from build123d import *
from build123d.topology import SkipClean

# Parameters (mm, degrees)
BASPROSKE_W         = 10
BASPROSKE_H         = 15
TOOTHCUT_DEPTH      = 24.452078799
TEETHCUTS_COUNT     = 28
TEETHCUTS_ANGLE     = 347.142857143
BORSKE_R            = 3.3
BORE_DEPTH          = 50.0000508
SKETCH_1_R          = 15
CUT_EXTRUDE_1_DEPTH = 6
CUT_EXTRUDE_2_DEPTH = 10
SKETCH_3_R          = 1.8
CUT_EXTRUDE_3_DEPTH = 10


with BuildPart() as part:
    # BasProSke → Base-Revolve (revolve)
    with BuildSketch(Plane(origin=(0, 0, 0), x_dir=(1, 0, 0), z_dir=(0, 1, 0)), mode=Mode.PRIVATE) as base_revolve_sk:
        with Locations((5, 7.5)):
            Rectangle(BASPROSKE_W, BASPROSKE_H)
    revolve(base_revolve_sk.sketch.rotate(Axis((-10, 0, 0), (1, 0, 0)), 180), axis=Axis((-10, 0, 0), (1, 0, 0)))

    # TooCutSke → ToothCut (cut, through all)
    with BuildSketch(Plane(origin=(0, 0, 0), x_dir=(0, 0, -1), z_dir=(1, 0, 0))):
        with BuildLine():
            ThreePointArc((0.471336039, 12.740284272), (0, 12.749), (-0.471336039, 12.740284272))
            ThreePointArc((-0.471336039, 12.740284272), (-0.81983923, 13.900763331), (-1.409805137, 14.959114099))
            ThreePointArc((-1.409805137, 14.959114099), (0, 15.0254), (1.409805137, 14.959114099))
            ThreePointArc((1.409805137, 14.959114099), (0.81983923, 13.900763331), (0.471336039, 12.740284272))
        make_face()
    toothcut = extrude(amount=TOOTHCUT_DEPTH, mode=Mode.SUBTRACT)

    # TeethCuts: ToothCut ×28 about axis
    teethcuts_axis = Axis((-10, 0, 0), (1, 0, 0))
    for i in range(1, TEETHCUTS_COUNT):
        add(toothcut.rotate(teethcuts_axis, i * TEETHCUTS_ANGLE / (TEETHCUTS_COUNT - 1)), mode=Mode.SUBTRACT)

    # BorSke → Bore (cut, symmetric)
    with BuildSketch(Plane(origin=(0, 0, 0), x_dir=(0, 0, -1), z_dir=(1, 0, 0))):
        with Locations(Location((0, 0, 0), (0, 0, 180))):
            Circle(BORSKE_R)
    extrude(amount=BORE_DEPTH, both=True, mode=Mode.SUBTRACT)

    # ｽｹｯﾁ1 → ｶｯﾄ - 押し出し1 (cut)
    with BuildSketch(Plane(origin=(10, 0, 0), x_dir=(0, 0, -1), z_dir=(1, 0, 0))):
        Circle(SKETCH_1_R)
    extrude(amount=-CUT_EXTRUDE_1_DEPTH, mode=Mode.SUBTRACT)

    # ｽｹｯﾁ2 → ｶｯﾄ - 押し出し2 (cut)
    with SkipClean():  # the faces are left unmerged after this step: merging them gives an invalid solid
        with BuildSketch(Plane.ZY):
            with BuildLine():
                Line((-12.525740882, -2.375461295), (-14.737321612, -2.794879553))
                ThreePointArc((-14.737321612, -2.794879553), (-6.004168657, 13.745906981), (12.065215177, 8.912383672))
                Line((12.065215177, 8.912383672), (10.254628553, 7.574931963))
                ThreePointArc((10.254628553, 7.574931963), (-5.10314308, 11.68310454), (-12.525740882, -2.375461295))
            make_face()
        extrude(amount=-CUT_EXTRUDE_2_DEPTH, mode=Mode.SUBTRACT)

    # ｽｹｯﾁ3 → ｶｯﾄ - 押し出し3 (cut)
    with SkipClean():  # the faces are left unmerged after this step: merging them gives an invalid solid
        with BuildSketch(Plane(origin=(4, 0, 0), x_dir=(0, 0, -1), z_dir=(1, 0, 0))):
            with Locations((-6.885831114, 1.259098832)):
                Circle(SKETCH_3_R)
            with Locations((1.259098832, 6.885831114)):
                Circle(SKETCH_3_R)
            with Locations((6.885831114, -1.259098832)):
                Circle(SKETCH_3_R)
            with Locations((-1.259098832, -6.885831114)):
                Circle(SKETCH_3_R)
        extrude(amount=-CUT_EXTRUDE_3_DEPTH, mode=Mode.SUBTRACT)


solid = part.part
Check sheet for the modelled part. Datum: model origin and axes. Units: mm. A direction names the side the tool comes from. Round coordinates to 2 decimals unless told otherwise and drop trailing zeros. Write each loop counter-clockwise with the first axis right and the second up, starting at its lowest first coordinate (ties: lowest second). Pieces come first, ordered by that corner, then holes. Notation, with made-up numbers: (5.25, 57.5) -> (37.25, 57.5) arc R17 ccw to (37.25, 87.5) -> close; hole circle Ø4 at (5.25, 19.25). An arc over 180 degrees is marked (long way). Answer as CSV lines item,"result". Start each with the question number.
1) Go/stop test with flat-tipped pins: P1, Ø1.5, axis at x = 1, y = -4.5, coming from the +Z side; P2, Ø3, axis at y = -1.26, z = -6.89, coming from the -X side; P3, Ø1.5, axis at x = 3, y = -0.5, coming from the +Z side. Record where each tip stops, or that it passes through.
2) Section check A-A on y = 0. Enter the section's corners in (x, z), and give its area (3 significant figures).
3) Release check for a two-part mould opening along Y. For faces 1 (the cylindrical face through (2, 2.3, 13.7)), 2 (the flat face through (4, -1, 4)), 3 (the cylindrical face through (1.972, -13.872, -0.808)) record: pulls with the +Y half, pulls with the -Y half, needs draft (parallel to the pull), parting line crosses it, or undercut.
4) Tool access check on faces 4 (the flat face through (0, -1, 4)), 5 (the cylindrical face through (2, -11.5, -5.5)), 6 (the cylindrical face through (1.972, -3.894, -13.372)), 7 (the cylindrical face through (1.97, -12.75, 0.01)), 8 (the cylindrical face through (1.97, -2.83, 12.43)). Record the directions out of +Z, -Z, +X, -X, +Y, -Y that give a thin tool (end or side, any length) a straight path to the whole face; none if there is none.
5) Section check C-C on x = 1.55. State how many separate pieces and enclosed holes the cut face has, and give its area (3 significant figures).
6) Material ranges on line 1 (Y direction, x = 2.1, z = -1.25); line 2 (Y direction, x = 1.3, z = 2.5); line 3 (Z direction, x = 3.5, y = -10.5), recorded low to high. Write a range as from..to.
Found:
1,P1,"stops at z = 14.25"
1,P2,"passes through"
1,P3,"stops at z = 14.72"
2,outline,"(0, -12.75) -> (4, -12.75) -> (4, -8.17) -> (0, -8.17) -> close; (0, -5.6) -> (4, -5.6) -> (4, -3.3) -> (0, -3.3) -> close; (0, 3.3) -> (4, 3.3) -> (4, 5.6) -> (0, 5.6) -> close; (0, 8.17) -> (4, 8.17) -> (4, 12.75) -> (0, 12.75) -> close"
2,area,"55.0 mm^2"
3,face 1,"undercut"
3,face 2,"needs draft"
3,face 3,"pulls with the -Y half"
4,face 4,"+Z, -Z, -X, +Y, -Y"
4,face 5,"+X, -X"
4,face 6,"-Z, +X, -X"
4,face 7,"+X, -X, -Y"
4,face 8,"+Z, +X, -X"
5,separate pieces,"1"
5,enclosed holes,"5"
5,area,"487 mm^2"
6,line 1,"y = -14.72..-3.05, 3.05..5.09, 8.69..12.69"
6,line 2,"y = -12.5..-8.19, -5.58..-2.15, 2.15..12.5"
6,line 3,"z = -10.71..-9.59, -7.7..7.7, 9.59..10.71"
